Part model, mm, in its own coordinate system. A direction names the side the tool comes from. Give positions to 0.01 mm unless a question says otherwise; leave off trailing zeros. Write each loop counter-clockwise with the first axis right and the second up, starting at its lowest first coordinate (ties: lowest second). Pieces come first, ordered by that corner, then holes. Notation, with made-up numbers: M 5.25,22.5 L 55.25,22.5 A23 ccw 55.25,41.5 Z; hole C 83,-21 d10. An arc over 180 degrees is marked long. Use a Markdown table: item, result.
```python
from build123d import *

# Parameters (mm, degrees)
F0_W        = 25.4
F0_H        = 19.05
F1_DEPTH    = 1.905
F3_DEPTH    = 12.7
F4_T1_DEPTH = 37.6967221242
F4_T3_DEPTH = 31.9335157919


# Not quite as in the source:
# - a fillet or chamfer that OpenCascade refuses, or shapes differently, is made with other operations: its cross-section is extruded or revolved along the edge and cut away or added


with BuildPart() as f1:
    # F0 (on Top) → F1 (new body)
    with BuildSketch(Plane.XY):
        Rectangle(F0_W, F0_H)
    extrude(amount=F1_DEPTH)

    # F2 (on Right) → F3 (join, symmetric)
    with BuildSketch(Plane.YZ):
        with BuildLine():
            ThreePointArc((-0.8833862371, 9.7538348994), (-4.3244369874, 6.4257362287), (-2.749630657, 1.905))
            Line((-2.749630657, 1.905), (2.749630657, 1.905))
            ThreePointArc((2.749630657, 1.905), (3.9987581366, 3.4563770351), (4.445, 5.3975))
            ThreePointArc((4.445, 5.3975), (3.4412698836, 8.2109829994), (0.8833862371, 9.7538348994))
            Line((0.8833862371, 9.7538348994), (0.8833862371, 8.4471317411))
            ThreePointArc((0.8833862371, 8.4471317411), (2.5382450929, 7.3048376336), (3.175, 5.3975))
            ThreePointArc((3.175, 5.3975), (-1.9073376336, 2.8592549071), (-0.8833862371, 8.4471317411))
            Line((-0.8833862371, 8.4471317411), (-0.8833862371, 9.7538348994))
        make_face()
    extrude(amount=F3_DEPTH, both=True)

    # F4: fillet of radius 2.54 on 4 edges, made by hand

    # F4_s2 → F4_t1 (cut)
    with BuildSketch(Plane.YZ.offset(-18.8483610621)):
        with BuildLine():
            ThreePointArc((-9.525, 0), (-8.6210815618, 1.3730463142), (-7.0656555752, 1.905))
            Line((-7.0656555752, 1.905), (-9.525, 1.905))
            Line((-9.525, 1.905), (-9.525, 0))
        make_face()
        with BuildLine():
            ThreePointArc((9.525, 0), (8.6210815618, 1.3730463142), (7.0656555752, 1.905))
            Line((7.0656555752, 1.905), (9.525, 1.905))
            Line((9.525, 1.905), (9.525, 0))
        make_face()
    extrude(amount=F4_T1_DEPTH, mode=Mode.SUBTRACT)

    # F4_s4 → F4_t3 (cut)
    with BuildSketch(Plane.YZ.offset(-15.9667578959)):
        with BuildLine():
            ThreePointArc((0.8833862371, 9.7538348994), (1.1966765002, 8.7408723938), (1.8962102849, 7.9440685845))
            ThreePointArc((1.8962102849, 7.9440685845), (1.4123764871, 8.2410572192), (0.8833862371, 8.4471317411))
            Line((0.8833862371, 8.4471317411), (0.8833862371, 9.7538348994))
        make_face()
        with BuildLine():
            ThreePointArc((-1.8962102849, 7.9440685845), (-1.1966765002, 8.7408723938), (-0.8833862371, 9.7538348994))
            Line((-0.8833862371, 9.7538348994), (-0.8833862371, 8.4471317411))
            ThreePointArc((-0.8833862371, 8.4471317411), (-1.4123764871, 8.2410572192), (-1.8962102849, 7.9440685845))
        make_face()
    extrude(amount=F4_T3_DEPTH, mode=Mode.SUBTRACT)


solid = f1.part
```
1. Tool access for faces 1 (the cylindrical face through (-0.178, -1.204, 8.728)), 2 (the flat face through (0, 5, 1.905)), 3 (the flat face through (0, -5, 1.905)), 4 (the cylindrical face through (-0.18, -8.64, 1.36)), 5 (the flat face through (-12.7, 0, 2)): list every direction of +Z, -Z, +X, -X, +Y, -Y with a clear straight run to the whole face (end or side of a thin tool).
Findings below:
| item | result |
|---|---|
| face 1 | +X, -X |
| face 2 | +X, -X, +Y |
| face 3 | +X, -X, -Y |
| face 4 | +Z, +X, -X, -Y |
| face 5 | +Z, -Z, -X, +Y, -Y |
2. Drop flat-ended pins along their axis: P1, Ø4, axis at x = 5, y = -3, coming from the +Z side; P2, Ø4, axis at x = 1, z = 6.5, coming from the +Y side (3 decimals); P3, Ø1.3, axis at x = -4, y = 4.5, coming from the +Z side. Give the stop position or say it passes through.
Findings below:
| item | result |
|---|---|
| P1 | z = 9.73 |
| P2 | y = 4.445 |
| P3 | z = 7.62 |
3. Cut at D-D, the plane y = 6. Give the cut face in (x, z) (3 decimals), then the cut area to 3 significant figures.
Findings below:
| item | result |
|---|---|
| outline | M -12.7,0 L 12.7,0 L 12.7,1.905 L -12.7,1.905 Z |
| area | 48.4 mm2 |
4. Cut at C-C, the plane y = 3.75. Give the cut face in (x, z) (3 decimals).
Findings below:
| item | result |
|---|---|
| outline | M -12.7,0 L 12.7,0 L 12.7,1.905 L -12.7,1.905 Z; M -12.7,3.011 L 12.7,3.011 L 12.7,7.784 L -12.7,7.784 Z |
5. Drill centre lines: L1, parallel to Z at x = -9.75, y = -6 (3 decimals); L2, parallel to Z at x = 10.25, y = 1.5; L3, parallel to Y at x = -1, z = 6.5. Where is each one in solid material? Low to high.
Findings below:
| item | result |
|---|---|
| L1 | 0 to 1.905 |
| L2 | 0 to 2.6, 8.31 to 9.58 |
| L3 | -4.31 to -2.98, 2.98 to 4.31 |
6. Two-plate mould, pull along Y, no slides. Class faces 6 (the flat face through (12.7, 0, 2)), 7 (the cylindrical face through (-0.18, 8.64, 1.36)), 8 (the cylindrical face through (-0.18, 1.19, 8.75)): released by +Y, released by -Y, zero draft, split by the parting line, or undercut.
Findings below:
| item | result |
|---|---|
| face 6 | zero draft |
| face 7 | released by +Y |
| face 8 | undercut |
7. Cut at A-A, the plane z = 3. Give the cut face in (x, y).
Findings below:
| item | result |
|---|---|
| outline | M -12.7,-3.74 L 12.7,-3.74 L 12.7,-2.08 L -12.7,-2.08 Z; M -12.7,2.08 L 12.7,2.08 L 12.7,3.74 L -12.7,3.74 Z |
